from build123d import *

# Parameters (mm, degrees)
SKETCH7_W               = 4.7625
SKETCH7_H               = 2.12122512
BOSS_EXTRUDE2_DEPTH     = 52.705
SKETCH8_W               = 2.12122512
SKETCH8_H               = 4.7625
BOSS_EXTRUDE3_DEPTH     = 52.705
BOSS_EXTRUDE4_DEPTH     = 52.705
CUT_EXTRUDE4_DEPTH      = 2.515570892
CUT_EXTRUDE4_DEPTH_BACK = 8.3025001
CUT_EXTRUDE5_DEPTH      = 8.3025001
CUT_EXTRUDE5_DEPTH_BACK = 2.500000148


with BuildPart() as part:
    # Sketch7 → Boss-Extrude2 (new body, symmetric)
    with BuildSketch(Plane.XY):
        with Locations((-4.92125, -2.560612608)):
            Rectangle(SKETCH7_W, SKETCH7_H)
    extrude(amount=BOSS_EXTRUDE2_DEPTH, both=True)

    # Sketch8 → Boss-Extrude3 (add, symmetric)
    with BuildSketch(Plane.XY):
        with Locations((-2.560612608, -4.92125)):
            Rectangle(SKETCH8_W, SKETCH8_H)
    extrude(amount=BOSS_EXTRUDE3_DEPTH, both=True)

    # Sketch11 → Boss-Extrude4 (add, symmetric)
    with BuildSketch(Plane.XY):
        with BuildLine():
            Line((-2.54, 1.500000048), (-2.54, -1.500000048))
            Line((-2.54, -1.500000048), (-7.3025, -1.500000048))
            Line((-7.3025, -1.500000048), (-7.3025, -3.621225168))
            Line((-7.3025, -3.621225168), (-5.866289198, -3.621225168))
            Line((-5.866289198, -3.621225168), (-3.621225168, -5.866289198))
            Line((-3.621225168, -5.866289198), (-3.621225168, -7.3025))
            Line((-3.621225168, -7.3025), (-1.500000048, -7.3025))
            Line((-1.500000048, -7.3025), (-1.500000048, -2.54))
            Line((-1.500000048, -2.54), (1.500000048, -2.54))
            add(Edge.make_bspline(
                [(-2.54, 1.500000048), (-1.295649087, 1.635512934), (-0.042467258, 0.473225958), (1.297713539, -0.292226779), (1.263724591, -2.340394541), (1.500000048, -2.54)],
                knots=[0, 0, 0, 0, 0.496686972, 0.741346965, 0.899739924, 0.899739924, 0.899739924, 0.899739924], degree=3))
        make_face()
    extrude(amount=BOSS_EXTRUDE4_DEPTH, both=True)

    # Sketch14 → Cut-Extrude4 (cut, two sides)
    with BuildSketch(Plane(origin=(0, 0, 0), x_dir=(1, 0, 0), z_dir=(0, 1, 0))) as cut_extrude4_sk:
        Polygon((-7.3025, -42.2275), (-7.3025, -56.8325), (7.3025, -56.8325), align=None)
        Polygon((-7.3025, 42.2275), (7.3025, 56.8325), (-7.3025, 56.8325), align=None)
    extrude(amount=CUT_EXTRUDE4_DEPTH, mode=Mode.SUBTRACT)
    extrude(cut_extrude4_sk.sketch, amount=-CUT_EXTRUDE4_DEPTH_BACK, mode=Mode.SUBTRACT)

    # Sketch17 → Cut-Extrude5 (cut, two sides)
    with BuildSketch(Plane(origin=(0, 0, 0), x_dir=(0, -1, 0), z_dir=(-1, 0, 0))) as cut_extrude5_sk:
        Polygon((7.3025, 56.8325), (7.3025, 42.2275), (-7.3025, 56.8325), align=None)
        Polygon((7.3025, -42.2275), (-7.3025, -56.8325), (7.3025, -56.8325), align=None)
    extrude(amount=CUT_EXTRUDE5_DEPTH, mode=Mode.SUBTRACT)
    extrude(cut_extrude5_sk.sketch, amount=-CUT_EXTRUDE5_DEPTH_BACK, mode=Mode.SUBTRACT)


solid = part.part
The model under review builds one solid part; all positions refer to its coordinate system, in mm. A direction names the side the tool comes from. Give positions to 0.01 mm unless a question says otherwise; leave off trailing zeros. One line per question, with ' | ' between items. Start each with the question number.
Item 1: For faces 1 (the flat face through (0, -2.54, 1)), 2 (the flat face through (-3.48, -1.86, 46.05)), 3 (the flat face through (-2.54, 0, 1)), list the 3-axis set-ups (+Z, -Z, +X, -X, +Y, -Y) from which the entire face can be reached by the end or side of a thin tool; tool diameter is ignored.
Item 2: For pin 1 (2.5 mm diameter, centred on y = -4.5, z = 6.5, fed in from +X); pin 2 (1.5 mm diameter, centred on y = 0.5, z = 15.5, fed in from -X); pin 3 (0.7 mm diameter, centred on x = -6.5, z = 3, fed in from -Y), all flat-tipped, find the tip position at first contact; note any pin that passes through.
Item 3: Wall thickness on line 1 (Y direction, x = -4.75, z = -25); line 2 (Y direction, x = -3, z = 19.5); line 3 (X direction, y = -6.25, z = 11): over which ranges is each line inside the solid? List them lowest first. Write a range as from..to.
Results found:
1) face 1: +Z, -Z, +X, -Y | face 2: +Z, -X, +Y, -Y | face 3: +Z, -Z, -X, +Y
2) pin 1: stops at x = -1.5 | pin 2: stops at x = -2.54 | pin 3: stops at y = -3.62
3) line 1: y = -4.74..-1.5 | line 2: y = -7.3..-1.5 | line 3: x = -3.62..-1.5
